Here's the drawing with two shaded views (mm, measured from the low corner). I have some questions. Coordinates: 2 decimals unless noted, no trailing zeros. Write each loop counter-clockwise with the first axis right and the second up, starting at its lowest first coordinate (ties: lowest second). Pieces come first, ordered by that corner, then holes.
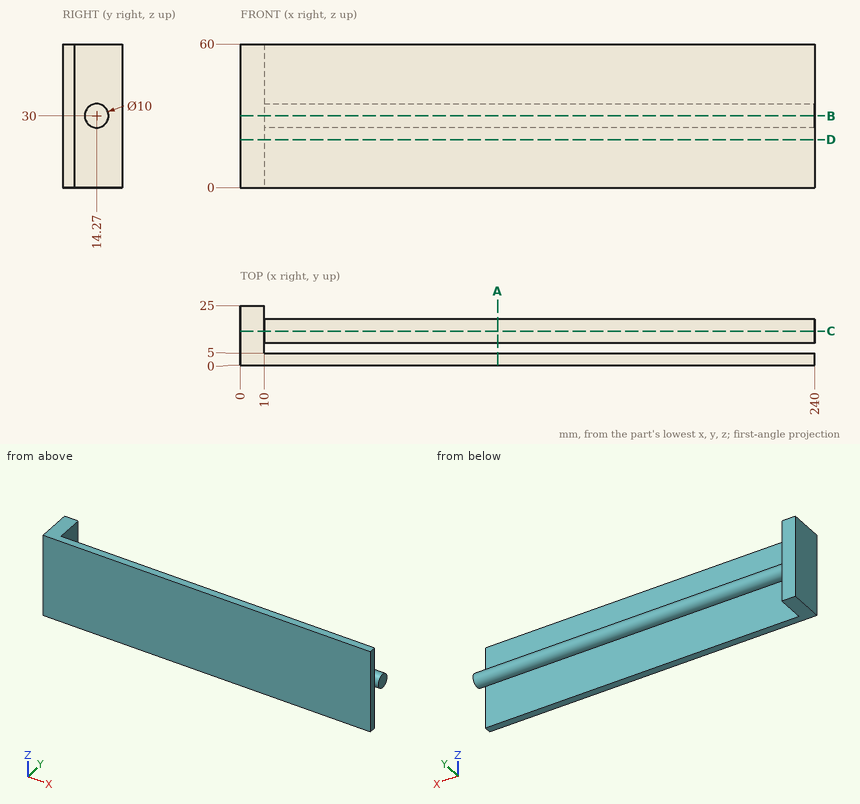
1. I want a section at D-D on z = 20. Please give me the cut outline in (x, y), plus the area to 3 significant figures.
Verdict:
outline: (0, 0) - (240, 0) - (240, 5) - (10, 5) - (10, 25) - (0, 25) - close
area: 1,400 mm2
2. I want a section at B-B on z = 30. Please give me the cut outline in (x, y), plus the area to 3 significant figures.
Verdict:
outline: (0, 0) - (240, 0) - (240, 5) - (10, 5) - (10, 9.27) - (240, 9.27) - (240, 19.27) - (10, 19.27) - (10, 25) - (0, 25) - close
area: 3,700 mm2
3. Please list where these lines run through material, in increasing order: line 1 along Y through (x, z) = (153.5, 8.5); line 2 along X through (y, z) = (10, 25); line 3 along Y through (x, z) = (134, 30.5).
Verdict:
line 1: y = 0 to 5
line 2: x = 0 to 10
line 3: y = 0 to 5, 9.3 to 19.24
4. For pin 1 (4 mm diameter, centred on x = 47.5, z = 47, fed in from +Y); pin 2 (8 mm diameter, centred on x = 43.5, y = 17.5, fed in from +Z); pin 3 (10 mm diameter, centred on y = 14.5, z = 41.5, fed in from +X), each with a flat end and sliding along its axis, tell me the tip position at first contact or that it passes through.
Verdict:
pin 1: stops at y = 5
pin 2: stops at z = 35
pin 3: stops at x = 10
5. I want a section at A-A on x = 107.5. Please give me the cut outline in (y, z), plus the area to 3 significant figures.
Verdict:
outline: (0, 0) - (5, 0) - (5, 60) - (0, 60) - close; circle Ø10 at (14.27, 30)
area: 379 mm2
6. I want a section at C-C on y = 14.27. Please give me the cut outline in (x, z), plus the area to 3 significant figures.
Verdict:
outline: (0, 0) - (10, 0) - (10, 25) - (240, 25) - (240, 35) - (10, 35) - (10, 60) - (0, 60) - close
area: 2,900 mm2
